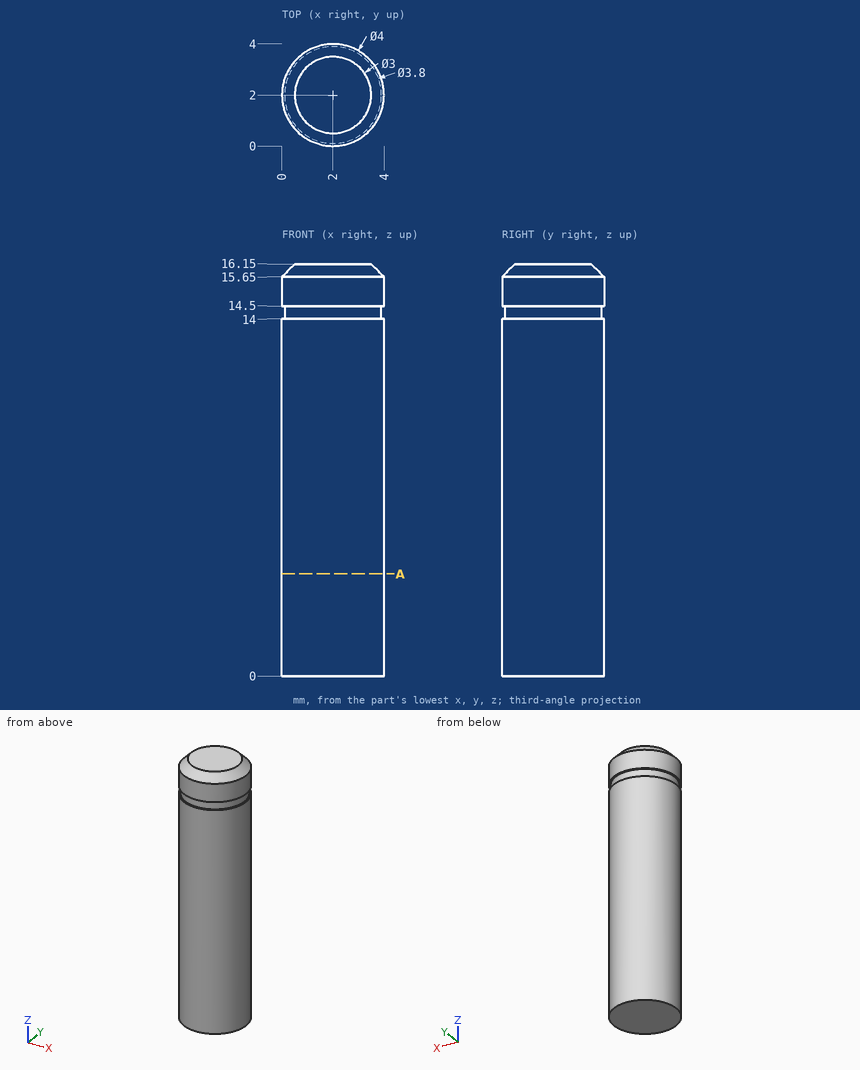
Study the drawing (mm; zero at the part's minimum x, y, z) and answer. Give positions to 0.01 mm unless a question says otherwise; leave off trailing zeros. Loops run counter-clockwise (first coordinate to the right, second up) from the corner with the lowest first, then second, coordinate; pieces in that order, holes last. Notation, with made-up numbers: M 5,25 L 44,25 A33 cw 44,59 Z; hole C 79,-24.5 d11. An arc over 180 degrees is marked long. One line per item, written item: value.
1. Each of these flat-tipped pins is pushed along its axis until it touches: P1, Ø1, axis at x = 3, z = 10, coming from the +Y side; P2, Ø2, axis at y = 2.5, z = 13.5, coming from the -X side. Where does it stop, or does it pass through?
Found:
P1: y = 3.94
P2: x = 0
2. Find the intervals of material crossed by probe 1 along Y at (x, z) = (2.1, 9.25); probe 2 along Y at (x, z) = (1, 3.75); probe 3 along X at (y, z) = (1.6, 11.25), in increasing order.
Found:
probe 1: 0 to 4
probe 2: 0.27 to 3.73
probe 3: 0.04 to 3.96
3. Section A-A on z = 4 is taken. Determine the outline of the cut face in (x, y), plus the area to 3 significant figures.
Found:
outline: C 2,2 d4
area: 12.6 mm^2
